from build123d import *

# Parameters (mm, degrees)
CROQUIS3_R              = 2.5
SALIENTE_EXTRUIR1_DEPTH = 2.5
CROQUIS4_R              = 1
SALIENTE_EXTRUIR2_DEPTH = 5
CROQUIS6_R              = 2.760916645
CORTAR_EXTRUIR1_DEPTH   = 35
SALIENTE_EXTRUIR3_START = -1
CROQUIS7_R              = 14
SALIENTE_EXTRUIR3_DEPTH = 1
CROQUIS8_R              = 15.075481364
SALIENTE_EXTRUIR4_DEPTH = 5.5
CROQUIS9_R              = 15.022760534
SALIENTE_EXTRUIR5_DEPTH = 2


# Read off the part's stored shape, not the designer's step: Vaciado1
with BuildPart() as part:
    # Croquis2 → Revolución1 (revolve)
    with BuildSketch(Plane(origin=(0, 0, 0), x_dir=(0, 0, -1), z_dir=(1, 0, 0))):
        Polygon((0, -9.212888184), (15, -9.212888184), (15, 8.787111816), (4.400455902, 19.788614132), (0, 19.788614132), align=None)
    revolve(axis=Axis((0, -10.664729222, 0), (0, 1, 0)))

    # Croquis3 → Saliente-Extruir1 (add)
    with BuildSketch(Plane(origin=(0, 19.788614132, 0), x_dir=(1, 0, 0), z_dir=(0, 1, 0))):
        with Locations(Location((0, 0, 0), (0, 0, 270))):
            Circle(CROQUIS3_R)
    extrude(amount=SALIENTE_EXTRUIR1_DEPTH)

    # Croquis4 → Saliente-Extruir2 (add)
    with BuildSketch(Plane(origin=(0, 22.288614132, 0), x_dir=(1, 0, 0), z_dir=(0, 1, 0))):
        with Locations(Location((0, 0, 0), (0, 0, 270))):
            Circle(CROQUIS4_R)
    extrude(amount=SALIENTE_EXTRUIR2_DEPTH)

    # Vaciado1 outline → Vaciado1 (revolve, cut)
    with BuildSketch(Plane.XY):
        Polygon((14, -9.212888184), (14, 8.383755945), (3.975300644, 18.788614132), (1.5, 18.788614132), (1.5, 21.288614132), (0, 21.288614132), (0, -9.212888184), align=None)
    revolve(axis=Axis((0, 0, 0), (0, 1, 0)), mode=Mode.SUBTRACT)

    # Croquis6 → Cortar-Extruir1 (cut)
    with BuildSketch(Plane(origin=(0, 19.788614132, 0), x_dir=(1, 0, 0), z_dir=(0, 1, 0))):
        with Locations(Location((0, -9.487911963, 0), (0, 0, 168.367798153))):
            Circle(CROQUIS6_R)
        with Locations(Location((-9.487911963, 0, 0), (0, 0, 155.446542586))):
            Circle(CROQUIS6_R)
        with Locations(Location((0, 9.487911963, 0), (0, 0, 270.000000733))):
            Circle(CROQUIS6_R)
        with Locations(Location((9.487911963, 0, 0), (0, 0, 99.378357768))):
            Circle(CROQUIS6_R)
    extrude(amount=-CORTAR_EXTRUIR1_DEPTH, mode=Mode.SUBTRACT)

    # Croquis7 → Saliente-Extruir3 (add)
    with BuildSketch(Plane.XZ.offset(9.212888184).offset(SALIENTE_EXTRUIR3_START)):
        with Locations(Location((0, 0, 0), (0, 0, 270))):
            Circle(CROQUIS7_R)
    extrude(amount=SALIENTE_EXTRUIR3_DEPTH)

    # Croquis8 → Saliente-Extruir4 (add, symmetric)
    with BuildSketch(Plane(origin=(0, 0, 0), x_dir=(1, 0, 0), z_dir=(0, 1, 0))):
        with Locations(Location((0, 0, 0), (0, 0, 270))):
            Circle(CROQUIS8_R)
    extrude(amount=SALIENTE_EXTRUIR4_DEPTH, both=True)

    # Croquis9 → Saliente-Extruir5 (add)
    with BuildSketch(Plane.XZ.offset(5.5)):
        with Locations(Location((0, 0, 0), (0, 0, 90))):
            Circle(CROQUIS9_R)
    extrude(amount=SALIENTE_EXTRUIR5_DEPTH)


solid = part.part
For this review, take the finished solid that the model builds, in its own axes (mm). A direction names the side the tool comes from. Give positions to 0.01 mm unless a question says otherwise; leave off trailing zeros. Loops run counter-clockwise (first coordinate to the right, second up) from the corner with the lowest first, then second, coordinate; pieces in that order, holes last. Notation, with made-up numbers: M 10.25,57.25 L 25.25,57.25 A15 ccw 25.25,64.25 Z; hole C -8,-25 d2. An arc over 180 degrees is marked long. Put each result on its own line as item: value. Start each with the question number.
(1) Add section B-B, the plane x = -2. Give the number of separate pieces and of enclosed holes in the cut face, then the cut area to 3 significant figures.
(2) Machinability: for faces 1 (the cylindrical face through (8.764, 13.804, -2.664)), 2 (the flat face through (0, -8.213, 0)), 3 (the cylindrical face through (-0.66, -8.344, 14.985)), which of the approach directions +Z, -Z, +X, -X, +Y, -Y give a long, thin tool a straight path to every point of the face, cutting with its end or side? Answer none if there is none.
(3) Add section D-D, the plane y = -5. Write out the cut boundary in (x, z), then the cut area to 3 significant figures.
(4) The part is to be moulded in two halves that separate along X. For faces 4 (the conical face through (4.122, 18.283, 1.709)), 5 (the flat face through (0, 5.5, 0)), 6 (the flat face through (2, 19.789, -2)), 7 (the cylindrical face through (14.666, -6.486, -3.257)), say which applies: +X half, -X half, draft (parallel to the pull), parting line (faces both ways), or undercut.
(5) For pin 1 (1 mm diameter, centred on y = 9, z = -3, fed in from +X); pin 2 (8 mm diameter, centred on y = 0.5, z = -10.5, fed in from -X); pin 3 (8 mm diameter, centred on x = 8, y = 20, fed in from +Z); pin 4 (1 mm diameter, centred on x = 5.5, y = 20.5, fed in from +Z), all flat-tipped, find the tip position at first contact; note any pin that passes through.
(6) Wall thickness on L1, parallel to Y at x = 0.5, z = 1; L2, parallel to Y at x = -1, z = 2; L3, parallel to Z at x = 0, y = -8.1: over which ranges is each line inside the solid? List them lowest first.
(7) Add section A-A, the plane y = 11. Write out the cut boundary in (x, z), then the cut area to 3 significant figures.
Result:
1. separate pieces: 2
1. enclosed holes: 1
1. area: 460 mm^2
2. face 1: +Y
2. face 2: none
2. face 3: -Y
3. outline: C 0,0 d30.15
3. area: 714 mm^2
4. face 4: undercut
4. face 5: undercut
4. face 6: draft
4. face 7: parting line
5. pin 1: stops at x = 14.78
5. pin 2: stops at x = -13.6
5. pin 3: stops at z = 4.65
5. pin 4: passes through
6. L1: y = -9.21 to -8.21, -7.5 to 5.5, 21.29 to 22.29
6. L2: y = -9.21 to -8.21, -7.5 to 5.5, 18.79 to 22.29
6. L3: z = -15 to -14, 14 to 15
7. outline: C 0,0 d25.74; hole M -11.29,-2.09 A11.48 ccw -2.09,-11.29 A2.76 ccw 2.09,-11.29 A11.48 ccw 11.29,-2.09 A2.76 ccw 11.29,2.09 A11.48 ccw 2.09,11.29 A2.76 ccw -2.09,11.29 A11.48 ccw -11.29,2.09 A2.76 ccw Z
7. area: 97.2 mm^2
